from build123d import *

# Parameters (mm, degrees)
F1_R     = 2.38125
F2_DEPTH = 5.2


with BuildPart() as f2:
    # F1 (on Top) → F2 (new body)
    with BuildSketch(Plane.XY):
        with BuildLine():
            Line((-250, 6.35), (-250, 250))
            Line((-250, 250), (0, 250))
            Line((0, 250), (0, 288.1))
            Line((0, 288.1), (-262.7, 288.1))
            ThreePointArc((-262.7, 288.1), (-280.660512, 280.660512), (-288.1, 262.7))
            Line((-288.1, 262.7), (-288.1, 0))
            Line((-288.1, 0), (-269.05, 0))
            Line((-269.05, 0), (-269.05, 3.175))
            ThreePointArc((-269.05, 3.175), (-268.120064, 5.420064), (-265.875, 6.35))
            Line((-265.875, 6.35), (-250, 6.35))
        make_face()
        with Locations((-275.4, 12.7)):
            Circle(F1_R, mode=Mode.SUBTRACT)
        with Locations((-262.7, 96.033333)):
            Circle(F1_R, mode=Mode.SUBTRACT)
        with Locations((-275.4, 179.366667)):
            Circle(F1_R, mode=Mode.SUBTRACT)
        with Locations((-262.7, 262.7)):
            Circle(F1_R, mode=Mode.SUBTRACT)
        with Locations((-179.366667, 275.4)):
            Circle(F1_R, mode=Mode.SUBTRACT)
        with Locations((-96.033333, 262.7)):
            Circle(F1_R, mode=Mode.SUBTRACT)
        with Locations((-12.7, 275.4)):
            Circle(F1_R, mode=Mode.SUBTRACT)
    extrude(amount=F2_DEPTH)


solid = f2.part
Source: CAD feature listing. Evaluate the final solid. Frame: model axes, mm. Round coordinates to 2 decimals unless told otherwise and drop trailing zeros. Loops run counter-clockwise (first coordinate to the right, second up) from the corner with the lowest first, then second, coordinate; pieces in that order, holes last.
Q1. Ray query, line 1 (X direction, y = 275.4, z = 2.75); line 2 (Y direction, x = -262.7, z = 3.15); line 3 (Y direction, x = -12.7, z = 2.55). Return the intervals inside material, ascending.
Q2. Section C-C, the plane y = 76.5. Return loops of the section in (x, z).
Q3. First-contact query: P1, Ø1.5, axis at x = -258, z = 2.5, coming from the -Y side; P2, Ø1.6, axis at y = 154, z = 1.5, coming from the +X side; P3, Ø7.5, axis at x = -179.37, y = 275.4, coming from the -Z side; P4, Ø1, axis at x = -234.5, z = 2, coming from the -Y side. Flat tips, straight axial feed; report the tip coordinate or a pass-through.
Q4. Section B-B, the plane x = -207. Return loops of the section in (y, z).
Q5. Section A-A, the plane z = 3.5. State how many separate pieces and enclosed holes the cut face has, plus the area to 3 significant figures.
Solutions:
1. line 1: x = -284.7 to -181.75, -176.99 to -15.08, -10.32 to 0
1. line 2: y = 6.35 to 93.65, 98.41 to 260.32, 265.08 to 288.1
1. line 3: y = 250 to 273.02, 277.78 to 288.1
2. outline: (-288.1, 0) - (-250, 0) - (-250, 5.2) - (-288.1, 5.2) - close
3. P1: stops at y = 6.35
3. P2: stops at x = -250
3. P3: stops at z = 0
3. P4: stops at y = 250
4. outline: (250, 0) - (288.1, 0) - (288.1, 5.2) - (250, 5.2) - close
5. separate pieces: 1
5. enclosed holes: 7
5. area: 20,100 mm2
